Read the model definition and answer for the solid it produces. Units are mm, in the model's axes. A direction names the side the tool comes from. Round coordinates to 2 decimals unless told otherwise and drop trailing zeros. Order: outer loops, then holes, each group sorted by start corner. A loop starts at its lowest first (then second) coordinate and runs counter-clockwise, first axis right, second up. Notation, with made-up numbers: (15, 10.25) -> (27, 10.25) arc R34 cw to (27, 41.25) -> close; hole circle Ø11 at (69.25, -6.75). An arc over 180 degrees is marked (long way). Use a Markdown table: item, result. Add a question column.
1. The mould has two halves that part along Z. Classify faces 1 (the face through (340.5, 19.257, -2.3)), 2 (the face through (331.294, -0.097, 2.307)), 3 (the face through (332.185, -16.864, 10.752)): +Z half, -Z half, draft (parallel to the pull), parting line (faces both ways), or undercut.
2. Given pin 1 (5 mm diameter, centred on x = 166, y = 14, fed in from -Z); pin 2 (5 mm diameter, centred on x = 311, z = -15.5, fed in from -Y); pin 3 (6 mm diameter, centred on x = 117.5, z = 0, fed in from +Y), each flat-ended and moving along its own axis, determine where each tip first touches the part or whether it passes through.
3. For faces 4 (the face through (210, -10, -8)), 5 (the face through (355, -1, 0)), determine the directions among +Z, -Z, +X, -X, +Y, -Y from which every point of the face is accessible in a straight line to the end or side of a thin tool.
4. Section B-B, the plane y = 0 is taken. Give the vertices of the cut face in (x, z), then the cut area to 3 significant figures.
5. Section D-D, the plane x = 89 is taken. Give the vertices of the cut face in (y, z), then the cut area to 3 significant figures.
6. Section C-C, the plane x = 278 is taken. Give the vertices of the cut face in (y, z), then the cut area to 3 significant figures.
7. Consider L1, parallel to X at y = 0, z = 0; L2, parallel to Y at x = 300.5, z = 0.5; L3, parallel to Z at x = 338.5, y = -4.5. Determine where each line is inside the solid, lowest interval first. Write a range as [from, to].
8. Section A-A, the plane z = 0 is taken. Give the vertices of the cut face in (x, y).
```python
from build123d import *

# Parameters (mm, degrees)
CROQUIS2_R                 = 12.5
SALIENTE_EXTRUIR1_DEPTH    = 210
CROQUIS4_R                 = 16.25
SALIENTE_EXTRUIR2_DEPTH    = 100
CROQUIS5_R                 = 20
SALIENTE_EXTRUIR3_DEPTH    = 45
CROQUIS6_W                 = 10.799694728
CROQUIS6_H                 = 1.485501512
CORTAR_EXTRUIR1_DEPTH      = 38
CORTAR_EXTRUIR2_REACH      = 359.724
CORTAR_EXTRUIR2_END_RADIUS = 20
CROQUIS8_R                 = 5


with BuildPart() as part:
    # Croquis2 → Saliente-Extruir1 (new body)
    with BuildSketch(Plane(origin=(0, 0, 0), x_dir=(0, 0, -1), z_dir=(1, 0, 0))):
        Circle(CROQUIS2_R)
    extrude(amount=SALIENTE_EXTRUIR1_DEPTH)

    # Croquis4 → Saliente-Extruir2 (add)
    with BuildSketch(Plane(origin=(210, 0, 0), x_dir=(0, 0, -1), z_dir=(1, 0, 0))):
        Circle(CROQUIS4_R)
    extrude(amount=SALIENTE_EXTRUIR2_DEPTH)

    # Croquis5 → Saliente-Extruir3 (add)
    with BuildSketch(Plane(origin=(310, 0, 0), x_dir=(0, 0, -1), z_dir=(1, 0, 0))):
        with Locations(Location((0, 0, 0), (0, 0, 180))):
            Circle(CROQUIS5_R)
    extrude(amount=SALIENTE_EXTRUIR3_DEPTH)

    # Croquis6 → Cortar-Extruir1 (cut)
    with BuildSketch(Plane(origin=(355, 0, 0), x_dir=(0, 0, -1), z_dir=(1, 0, 0))):
        with Locations((0, 20)):
            Rectangle(CROQUIS6_W, CROQUIS6_H)
    extrude(amount=-CORTAR_EXTRUIR1_DEPTH, mode=Mode.SUBTRACT)

    # Cortar-Extruir2: up to this cylinder (the profile starts inside it)
    cortar_extruir2_end = Plane(origin=(335.730152, 0, 0), z_dir=(-1, 0, 0)) * Cylinder(CORTAR_EXTRUIR2_END_RADIUS, 760.448, mode=Mode.PRIVATE)
    # Croquis8 → Cortar-Extruir2 (cut, up to the surface)
    with BuildSketch(Plane(origin=(0, 19.257249244, 0), x_dir=(1, 0, 0), z_dir=(0, 1, 0)), mode=Mode.PRIVATE) as cortar_extruir2_sk1:
        with Locations(Location((335.730152453, 0, 0), (0, 0, 270))):
            Circle(CROQUIS8_R)
    cortar_extruir2_tool1 = extrude(cortar_extruir2_sk1.sketch, amount=-CORTAR_EXTRUIR2_REACH, mode=Mode.PRIVATE) & cortar_extruir2_end
    add(cortar_extruir2_tool1.solids().sort_by_distance((335.730152, 19.257249, 0))[0], mode=Mode.SUBTRACT)


solid = part.part
```
Verdict:
| question | item | result |
|---|---|---|
| 1 | face 1 | draft |
| 1 | face 2 | undercut |
| 1 | face 3 | parting line |
| 2 | pin 1 | stops at z = -4.9 |
| 2 | pin 2 | stops at y = -15.2 |
| 2 | pin 3 | stops at y = 12.5 |
| 3 | face 4 | -X |
| 3 | face 5 | +Z, -Z, +X, +Y, -Y |
| 4 | outline | (0, -12.5) -> (210, -12.5) -> (210, -16.25) -> (310, -16.25) -> (310, -20) -> (355, -20) -> (355, 20) -> (310, 20) -> (310, 16.25) -> (210, 16.25) -> (210, 12.5) -> (0, 12.5) -> close; hole circle Ø10 at (335.73, 0) |
| 4 | area | 10,200 mm2 |
| 5 | outline | circle Ø25 at (0, 0) |
| 5 | area | 491 mm2 |
| 6 | outline | circle Ø32.5 at (0, 0) |
| 6 | area | 830 mm2 |
| 7 | L1 | x = [0, 330.73], [340.73, 355] |
| 7 | L2 | y = [-16.24, 16.24] |
| 7 | L3 | z = [-19.49, -4.16], [4.16, 19.49] |
| 8 | outline | (0, -12.5) -> (210, -12.5) -> (210, -16.25) -> (310, -16.25) -> (310, -20) -> (330.73, -20) -> (330.73, 19.26) -> (317, 19.26) -> (317, 20) -> (310, 20) -> (310, 16.25) -> (210, 16.25) -> (210, 12.5) -> (0, 12.5) -> close; (340.73, -20) -> (355, -20) -> (355, 19.26) -> (340.73, 19.26) -> close |
